Here's how the part is built. I have some questions about the finished solid (model axes, mm). Give positions to 0.01 mm unless a question says otherwise; leave off trailing zeros. Loops run counter-clockwise (first coordinate to the right, second up) from the corner with the lowest first, then second, coordinate; pieces in that order, holes last. Notation, with made-up numbers: M -11,66 L 3,66 A35 ccw 3,99 Z; hole C -22.75,71 d10. An arc over 180 degrees is marked long. Answer as CSV lines item,"result". Start each with the question number.
Item 1: If I drill on line 1 along Y through (x, z) = (827.5, 2); line 2 along X through (y, z) = (287.5, 2); line 3 along Y through (x, z) = (70, 4.25), over which ranges is the centre line in solid material (lowest first)? Write a range as from..to.
Item 2: I want a section at B-B on y = 173. List the corners of the cut face in (x, z) for me.
Item 3: I want a section at A-A on x = 710.5. List the corners of the cut face in (y, z) for me.
Item 4: Will this pin go through, and if not, where does the flat tip stop? P1, Ø5.5, axis at x = 420, y = 12.5, coming from the +Z side.
Item 5: I want a section at C-C on y = 224. Give the number of separate pieces and of enclosed holes in the cut face, plus the area to 3 significant figures.
from build123d import *

# Parameters (mm, degrees)
SKETCH2_W           = 840
SKETCH2_H           = 300
BOSS_EXTRUDE1_DEPTH = 6.35
CUT_EXTRUDE1_DEPTH  = 6.35
SKETCH4_R           = 3.5
CUT_EXTRUDE2_DEPTH  = 892.98672776
SKETCH5_W           = 180
SKETCH5_H           = 127.5
CUT_EXTRUDE3_DEPTH  = 892.98672776
FILLET1_R           = 3.5


with BuildPart() as part:
    # Sketch2 → Boss-Extrude1 (new body)
    with BuildSketch(Plane.XY):
        with Locations((420, 150)):
            Rectangle(SKETCH2_W, SKETCH2_H)
    extrude(amount=BOSS_EXTRUDE1_DEPTH)

    # Sketch3 → Cut-Extrude1 (cut)
    with BuildSketch(Plane.XY.offset(6.35)):
        with BuildLine():
            Line((413.65, 210), (413.65, 260))
            ThreePointArc((413.65, 260), (420, 266.35), (426.35, 260))
            Line((426.35, 260), (426.35, 210))
            ThreePointArc((426.35, 210), (420, 203.65), (413.65, 210))
        make_face()
        with BuildLine():
            Line((451.35, 210), (451.35, 260))
            ThreePointArc((451.35, 260), (445, 266.35), (438.65, 260))
            Line((438.65, 260), (438.65, 210))
            ThreePointArc((438.65, 210), (445, 203.65), (451.35, 210))
        make_face()
        with BuildLine():
            Line((476.35, 210), (476.35, 260))
            ThreePointArc((476.35, 260), (470, 266.35), (463.65, 260))
            Line((463.65, 260), (463.65, 210))
            ThreePointArc((463.65, 210), (470, 203.65), (476.35, 210))
        make_face()
        with BuildLine():
            Line((501.35, 210), (501.35, 260))
            ThreePointArc((501.35, 260), (495, 266.35), (488.65, 260))
            Line((488.65, 260), (488.65, 210))
            ThreePointArc((488.65, 210), (495, 203.65), (501.35, 210))
        make_face()
        with BuildLine():
            Line((401.35, 210), (401.35, 260))
            ThreePointArc((401.35, 260), (395, 266.35), (388.65, 260))
            Line((388.65, 260), (388.65, 210))
            ThreePointArc((388.65, 210), (395, 203.65), (401.35, 210))
        make_face()
        with BuildLine():
            Line((376.35, 210), (376.35, 260))
            ThreePointArc((376.35, 260), (370, 266.35), (363.65, 260))
            Line((363.65, 260), (363.65, 210))
            ThreePointArc((363.65, 210), (370, 203.65), (376.35, 210))
        make_face()
        with BuildLine():
            Line((351.35, 210), (351.35, 260))
            ThreePointArc((351.35, 260), (345, 266.35), (338.65, 260))
            Line((338.65, 260), (338.65, 210))
            ThreePointArc((338.65, 210), (345, 203.65), (351.35, 210))
        make_face()
        with BuildLine():
            Line((326.35, 210), (326.35, 260))
            ThreePointArc((326.35, 260), (320, 266.35), (313.65, 260))
            Line((313.65, 260), (313.65, 210))
            ThreePointArc((313.65, 210), (320, 203.65), (326.35, 210))
        make_face()
        with BuildLine():
            Line((301.35, 210), (301.35, 260))
            ThreePointArc((301.35, 260), (295, 266.35), (288.65, 260))
            Line((288.65, 260), (288.65, 210))
            ThreePointArc((288.65, 210), (295, 203.65), (301.35, 210))
        make_face()
        with BuildLine():
            Line((276.35, 210), (276.35, 260))
            ThreePointArc((276.35, 260), (270, 266.35), (263.65, 260))
            Line((263.65, 260), (263.65, 210))
            ThreePointArc((263.65, 210), (270, 203.65), (276.35, 210))
        make_face()
        with BuildLine():
            Line((251.35, 210), (251.35, 260))
            ThreePointArc((251.35, 260), (245, 266.35), (238.65, 260))
            Line((238.65, 260), (238.65, 210))
            ThreePointArc((238.65, 210), (245, 203.65), (251.35, 210))
        make_face()
        with BuildLine():
            Line((226.35, 210), (226.35, 260))
            ThreePointArc((226.35, 260), (220, 266.35), (213.65, 260))
            Line((213.65, 260), (213.65, 210))
            ThreePointArc((213.65, 210), (220, 203.65), (226.35, 210))
        make_face()
        with BuildLine():
            Line((201.35, 210), (201.35, 260))
            ThreePointArc((201.35, 260), (195, 266.35), (188.65, 260))
            Line((188.65, 260), (188.65, 210))
            ThreePointArc((188.65, 210), (195, 203.65), (201.35, 210))
        make_face()
        with BuildLine():
            Line((176.35, 210), (176.35, 260))
            ThreePointArc((176.35, 260), (170, 266.35), (163.65, 260))
            Line((163.65, 260), (163.65, 210))
            ThreePointArc((163.65, 210), (170, 203.65), (176.35, 210))
        make_face()
        with BuildLine():
            Line((151.35, 210), (151.35, 260))
            ThreePointArc((151.35, 260), (145, 266.35), (138.65, 260))
            Line((138.65, 260), (138.65, 210))
            ThreePointArc((138.65, 210), (145, 203.65), (151.35, 210))
        make_face()
        with BuildLine():
            Line((126.35, 210), (126.35, 260))
            ThreePointArc((126.35, 260), (120, 266.35), (113.65, 260))
            Line((113.65, 260), (113.65, 210))
            ThreePointArc((113.65, 210), (120, 203.65), (126.35, 210))
        make_face()
        with BuildLine():
            Line((101.35, 210), (101.35, 260))
            ThreePointArc((101.35, 260), (95, 266.35), (88.65, 260))
            Line((88.65, 260), (88.65, 210))
            ThreePointArc((88.65, 210), (95, 203.65), (101.35, 210))
        make_face()
        with BuildLine():
            Line((76.35, 210), (76.35, 260))
            ThreePointArc((76.35, 260), (70, 266.35), (63.65, 260))
            Line((63.65, 260), (63.65, 210))
            ThreePointArc((63.65, 210), (70, 203.65), (76.35, 210))
        make_face()
        with BuildLine():
            Line((526.35, 210), (526.35, 260))
            ThreePointArc((526.35, 260), (520, 266.35), (513.65, 260))
            Line((513.65, 260), (513.65, 210))
            ThreePointArc((513.65, 210), (520, 203.65), (526.35, 210))
        make_face()
        with BuildLine():
            Line((551.35, 210), (551.35, 260))
            ThreePointArc((551.35, 260), (545, 266.35), (538.65, 260))
            Line((538.65, 260), (538.65, 210))
            ThreePointArc((538.65, 210), (545, 203.65), (551.35, 210))
        make_face()
    extrude(amount=-CUT_EXTRUDE1_DEPTH, mode=Mode.SUBTRACT)

    # Sketch4 → Cut-Extrude2 (cut, through all)
    with BuildSketch(Plane.XY.offset(6.35)):
        with Locations((420, 287.5)):
            Circle(SKETCH4_R)
        with Locations((770, 287.5)):
            Circle(SKETCH4_R)
        with Locations((70, 287.5)):
            Circle(SKETCH4_R)
        with Locations((12.5, 250)):
            Circle(SKETCH4_R)
        with Locations((12.5, 50)):
            Circle(SKETCH4_R)
        with Locations(Location((827.5, 50, 0), (0, 0, 180))):
            Circle(SKETCH4_R)
        with Locations(Location((827.5, 250, 0), (0, 0, 180))):
            Circle(SKETCH4_R)
        with Locations(Location((770, 12.5, 0), (0, 0, 180))):
            Circle(SKETCH4_R)
        with Locations(Location((420, 12.5, 0), (0, 0, 180))):
            Circle(SKETCH4_R)
        with Locations(Location((70, 12.5, 0), (0, 0, 180))):
            Circle(SKETCH4_R)
        with Locations((373.25, 12.5)):
            Circle(SKETCH4_R)
        with Locations((466.75, 12.5)):
            Circle(SKETCH4_R)
    extrude(amount=-CUT_EXTRUDE2_DEPTH, mode=Mode.SUBTRACT)

    # Sketch5 → Cut-Extrude3 (cut, through all)
    with BuildSketch(Plane.XY.offset(6.35)):
        with Locations((701, 187.5)):
            Rectangle(SKETCH5_W, SKETCH5_H)
    extrude(amount=-CUT_EXTRUDE3_DEPTH, mode=Mode.SUBTRACT)

    # Fillet1
    fillet1_edges = [part.edges().sort_by_distance(p)[0] for p in [
        (611, 123.75, 3.175),
        (611, 251.25, 3.175),
        (791, 251.25, 3.175),
        (791, 123.75, 3.175),
    ]]
    fillet(fillet1_edges, radius=FILLET1_R)


solid = part.part
Result:
1,line 1,"0..46.5, 53.5..246.5, 253.5..300"
1,line 2,"0..66.5, 73.5..416.5, 423.5..766.5, 773.5..840"
1,line 3,"0..9, 16..203.65, 266.35..284, 291..300"
2,outline,"M 0,0 L 611,0 L 611,6.35 L 0,6.35 Z; M 791,0 L 840,0 L 840,6.35 L 791,6.35 Z"
3,outline,"M 0,0 L 123.75,0 L 123.75,6.35 L 0,6.35 Z; M 251.25,0 L 300,0 L 300,6.35 L 251.25,6.35 Z"
4,P1,"through"
5,separate pieces,"22"
5,enclosed holes,"0"
5,area,"2,580 mm^2"
